Part model, mm, in its own coordinate system. Face numbers are marked on the shaded views. Round coordinates to 2 decimals unless told otherwise and drop trailing zeros. Loops run counter-clockwise (first coordinate to the right, second up) from the corner with the lowest first, then second, coordinate; pieces in that order, holes last. Notation, with made-up numbers: M 35.25,61 L 84.25,61 A25 cw 84.25,78 Z; hole C 38.5,88.25 d4. An arc over 180 degrees is marked long. Answer as CSV lines item,"result". Start each with the question number.
Item 1: Band-saw the part on A-A (y = -21.5). Give the cut face in (x, z), and give its area (3 significant figures).
Item 2: Wall check: line 1 (Z direction, x = -3.5, y = 1.5); line 2 (X direction, y = -14, z = 11.5). Give the ranges that are in metal, low to high.
Item 3: Drop flat-ended pins along their axis: pin 1 Ø2 at (y, z) = (18.5, 130.5) entering from -X; pin 2 Ø18.5 at (x, y) = (-1, 6) entering from +Z. Give the stop position or say it passes through.
Item 4: Band-saw the part on C-C (x = 10). Give the cut face in (y, z).
Item 5: Mould opens along Z. For the marked faces 1, 2 and 3 say: pulls with the +Z half, pulls with the -Z half, needs draft (parallel to the pull), parting line crosses it, or undercut.
Item 6: Band-saw the part on B-B (z = 52). Give the cut face in (x, y), and give its area (3 significant figures).
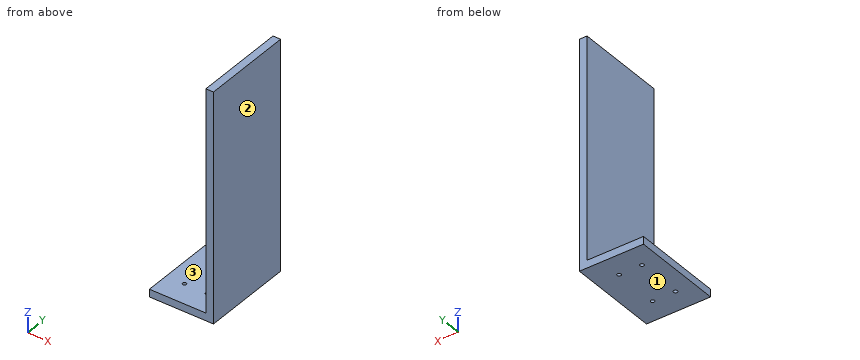
```python
from build123d import *

# Parameters (mm, degrees)
SKETCH_1_W         = 37
SKETCH_1_H         = 60
EXTRUDE_1_DEPTH    = 5
SKETCH_1_3_W       = 5
SKETCH_1_3_H       = 60
EXTRUDE_2_DEPTH    = 150
HOLE_WIZARD_M3_1_D = 2.5


with BuildPart() as part:
    # 草图1 → 凸台-拉伸1 (new body)
    with BuildSketch(Plane.XY):
        with Locations((-2.380104714, 0)):
            Rectangle(SKETCH_1_W, SKETCH_1_H)
    extrude(amount=EXTRUDE_1_DEPTH)

    # 草图1<3> → 凸台-拉伸2 (add)
    with BuildSketch(Plane.XY):
        with Locations((18.619895286, 0)):
            Rectangle(SKETCH_1_3_W, SKETCH_1_3_H)
    extrude(amount=EXTRUDE_2_DEPTH)

    # M3 螺纹孔的螺纹孔钻头1 (through all)
    with Locations(Plane(origin=(-8.880104714, 15, 5), x_dir=(1, 0, 0), z_dir=(0, 0, 1))):
        with Locations((0, 0), (15, 0)):
            hole_wizard_m3_1 = Hole(HOLE_WIZARD_M3_1_D / 2)

    # 镜向1: M3 螺纹孔的螺纹孔钻头1 across plane
    add(hole_wizard_m3_1.mirror(Plane.ZX), mode=Mode.SUBTRACT)


solid = part.part
```
Answer block:
1,outline,"M -20.88,0 L 21.12,0 L 21.12,150 L 16.12,150 L 16.12,5 L -20.88,5 Z"
1,area,"935 mm^2"
2,line 1,"z = 0 to 5"
2,line 2,"x = 16.12 to 21.12"
3,pin 1,"stops at x = 16.12"
3,pin 2,"stops at z = 5"
4,outline,"M -30,0 L 30,0 L 30,5 L -30,5 Z"
5,face 1,"pulls with the -Z half"
5,face 2,"needs draft"
5,face 3,"pulls with the +Z half"
6,outline,"M 16.12,-30 L 21.12,-30 L 21.12,30 L 16.12,30 Z"
6,area,"300 mm^2"
